from build123d import *

# Parameters (mm, degrees)
F0_R     = 3.175
F1_DEPTH = 12.7
F2_R     = 6.35
F3_DEPTH = 3.175
F5_DEPTH = 2.54
F6_R     = 3.175
F7_DEPTH = 12.7


with BuildPart() as f1:
    # F0 (on Top) → F1 (new body, symmetric)
    with BuildSketch(Plane.XY):
        Circle(F0_R)
    extrude(amount=F1_DEPTH, both=True)

    # F2 (on face) → F3 (join)
    with BuildSketch(Plane(origin=(0, 0, -12.7), x_dir=(1, 0, 0), z_dir=(0, 0, -1))):
        Circle(F2_R)
    extrude(amount=F3_DEPTH)

    # F4 (on face) → F5 (join)
    with BuildSketch(Plane.XY.offset(12.7)):
        with BuildLine():
            ThreePointArc((16.98045, -3.175), (19.225514, -2.245064), (20.15545, 0))
            ThreePointArc((20.15545, 0), (19.225514, 2.245064), (16.98045, 3.175))
            ThreePointArc((16.98045, 3.175), (13.80545, 0), (16.98045, -3.175))
        make_face()
        with BuildLine():
            ThreePointArc((16.98045, -3.175), (13.80545, 0), (16.98045, 3.175))
            Line((16.98045, 3.175), (0, 3.175))
            ThreePointArc((0, 3.175), (2.245064, 2.245064), (3.175, 0))
            ThreePointArc((3.175, 0), (2.245064, -2.245064), (0, -3.175))
            Line((0, -3.175), (16.98045, -3.175))
        make_face()
        with BuildLine():
            ThreePointArc((3.175, 0), (2.245064, 2.245064), (0, 3.175))
            ThreePointArc((0, 3.175), (-3.175, 0), (0, -3.175))
            ThreePointArc((0, -3.175), (2.245064, -2.245064), (3.175, 0))
        make_face()
    extrude(amount=F5_DEPTH)

    # F6 (on face) → F7 (join)
    with BuildSketch(Plane.XY.offset(15.24)):
        with Locations((16.98045, 0)):
            Circle(F6_R)
    extrude(amount=F7_DEPTH)


solid = f1.part
Could you check a few things on this model? Use its own coordinates, in mm. A direction names the side the tool comes from. Round coordinates to 2 decimals unless told otherwise and drop trailing zeros. Loops run counter-clockwise (first coordinate to the right, second up) from the corner with the lowest first, then second, coordinate; pieces in that order, holes last. Notation, with made-up numbers: (63.5, 56) -> (87.5, 56) arc R34 cw to (87.5, 88) -> close; hole circle Ø5 at (62, 39). An arc over 180 degrees is marked (long way). Use CSV: the item, a comma, the result in double quotes.
(1) Suppose I cut it at D-D on y = 5.75. Write out the boundary of the cut face in (x, z) (3 decimals).
Return value:
outline,"(-2.694, -15.875) -> (2.694, -15.875) -> (2.694, -12.7) -> (-2.694, -12.7) -> close"
(2) If we mould it in two halves opening along Z, with no side actions, what happens to faces 1 (the flat face through (-2, -3, -12.7)), 2 (the flat face through (0, 0, -15.875)), 3 (the flat face through (9, 3.175, 14)), 4 (the flat face through (17, 0, 27.94))? For each: +Z half, -Z half, draft (parallel to the pull), parting line (faces both ways), or undercut.
Return value:
face 1,"undercut"
face 2,"-Z half"
face 3,"draft"
face 4,"+Z half"
(3) For faces 5 (the flat face through (8, -3.175, 14)), 6 (the cylindrical face through (-1.38, 6.2, -14.27)), which set-ups out of +Z, -Z, +X, -X, +Y, -Y let a thin tool reach every point of the face, with its end or its side?
Return value:
face 5,"+Z, +X, -X, -Y"
face 6,"-Z"
(4) If I drill on probe 1 along Z at (x, y) = (-1.5, 1.25) (3 decimals); probe 2 along Z at (x, y) = (13, 0); probe 3 along X at (y, z) = (-0.25, -2.5), over which ranges is the centre line in solid material (lowest first)? Write a range as [from, to].
Return value:
probe 1,"z = [-15.875, 15.24]"
probe 2,"z = [12.7, 15.24]"
probe 3,"x = [-3.17, 3.17]"
(5) Suppose I cut it at C-C on x = 0.5. Write out the boundary of the cut face in (y, z) (3 decimals).
Return value:
outline,"(-6.33, -15.875) -> (6.33, -15.875) -> (6.33, -12.7) -> (3.135, -12.7) -> (3.135, 12.7) -> (3.175, 12.7) -> (3.175, 15.24) -> (-3.175, 15.24) -> (-3.175, 12.7) -> (-3.135, 12.7) -> (-3.135, -12.7) -> (-6.33, -12.7) -> close"
(6) Will these pins go through, and if not, where does the flat tip stop? pin 1 Ø1.5 at (x, z) = (1.5, 8.5) entering from -Y; pin 2 Ø1.3 at (x, z) = (9.5, 13.5) entering from +Y (3 decimals); pin 3 Ø3 at (x, y) = (10, 0.5) entering from +Z; pin 4 Ø1 at (x, y) = (6.5, 4.5) entering from -Z.
Return value:
pin 1,"stops at y = -3.09"
pin 2,"stops at y = 3.175"
pin 3,"stops at z = 15.24"
pin 4,"passes through"
(7) Suppose I cut it at B-B on z = -11. Write out the boundary of the cut face in (x, y) (3 decimals).
Return value:
outline,"circle Ø6.35 at (0, 0)"
(8) Suppose I cut it at A-A on x = 5. Write out the boundary of the cut face in (y, z) (3 decimals).
Return value:
outline,"(-3.914, -15.875) -> (3.914, -15.875) -> (3.914, -12.7) -> (-3.914, -12.7) -> close; (-3.175, 12.7) -> (3.175, 12.7) -> (3.175, 15.24) -> (-3.175, 15.24) -> close"
